Autodesk Inventor part; units mm, degrees
ref_plane "YZ Plane" through (0, 0, 0) normal (1, 0, 0) x (0, 1, 0)
ref_plane "XZ Plane" through (0, 0, 0) normal (0, 1, 0) x (-1, 0, 0)
ref_plane "XY Plane" through (0, 0, 0) normal (0, 0, 1) x (1, 0, 0)
sketch "스케치1" plane through (0, 0, 0) normal (0, 0, 1) x (1, 0, 0)
  line L0 (-3, 27) -> (3, 27)
  line L1 (3, 27) -> (3, -27)
  line L2 (3, -27) -> (-3, -27)
  line L3 (-3, -27) -> (-3, 27)
  point P0 (0, 0)
  dimension "d0" = 6
  dimension "d1" = 54
  dimension "d3" = 3
  dimension "d4" = 27
extrude "돌출1" add sketch "스케치1" along normal blind 4
sketch "스케치2" plane through (0, 0, 4) normal (0, 0, 1) x (1, 0, 0)
  line L0 (3, 27) -> (-3, 27)
  line L1 (-3, 27) -> (-3, -27)
  line L2 (-3, -27) -> (3, -27)
  line L3 (3, -27) -> (3, 27)
  circle A0 centre (0, 24) radius 1.6
  circle A1 centre (0, -24) radius 1.6
  point P0 (0, 0)
  dimension "d7" = 3.2
  dimension "d8" = 3.2
  dimension "d9" = 3
  dimension "d10" = 3
  dimension "d11" = 3
  dimension "d12" = 3
extrude "돌출2" cut sketch "스케치2" against normal up to next contours A0 | A1
chamfer "모따기1" distance 2 angle 45 4 edges at (3, 27, 2) (-3, 27, 2) (-3, -27, 2) (3, -27, 2)
properties part number "큰모터서포터" material "알루미늄 6061"
Can you work these out from the model? Positions are in its coordinate system, mm. Give positions to 0.01 mm unless a question says otherwise; leave off trailing zeros. Loops run counter-clockwise (first coordinate to the right, second up) from the corner with the lowest first, then second, coordinate; pieces in that order, holes last. Notation, with made-up numbers: M 70,54.5 L 96,54.5 A22 cw 96,88.5 Z; hole C -9,41.5 d3. An arc over 180 degrees is marked long. Answer in a Markdown table with one row per item.
1. If I drill on line 1 along Y through (x, z) = (0, 1.3); line 2 along Y through (x, z) = (0.75, 2.35); line 3 along Y through (x, z) = (2.75, 3.3), over which ranges is the centre line in solid material (lowest first)?
Taken from the geometry:
| item | result |
|---|---|
| line 1 | y = -27 to -25.6, -22.4 to 22.4, 25.6 to 27 |
| line 2 | y = -27 to -25.41, -22.59 to 22.59, 25.41 to 27 |
| line 3 | y = -25.25 to 25.25 |
2. For pin 1 Ø2 at (x, y) = (2, -7) entering from -Z, with a flat end and sliding along its axis, tell me the tip position at first contact or that it passes through.
Taken from the geometry:
| item | result |
|---|---|
| pin 1 | stops at z = 0 |
3. Suppose I cut it at A-A on x = 0. Write out the boundary of the cut face in (y, z), plus the area to 3 significant figures.
Taken from the geometry:
| item | result |
|---|---|
| outline | M -27,0 L -25.6,0 L -25.6,4 L -27,4 Z; M -22.4,0 L 22.4,0 L 22.4,4 L -22.4,4 Z; M 25.6,0 L 27,0 L 27,4 L 25.6,4 Z |
| area | 190 mm² |
4. Thinking about a two-plate mould opening in X: for faces 1 (the cylindrical face through (-0.208, 25.586, 2.028)), 2 (the flat face through (0, 0, 0)), 3 (the flat face through (2, 26, 2)), which applies, released by +X, released by -X, zero draft, split by the parting line, or undercut?
Taken from the geometry:
| item | result |
|---|---|
| face 1 | undercut |
| face 2 | zero draft |
| face 3 | released by +X |
5. Suppose I cut it at D-D on x = 2.3. Write out the boundary of the cut face in (y, z).
Taken from the geometry:
| item | result |
|---|---|
| outline | M -25.7,0 L 25.7,0 L 25.7,4 L -25.7,4 Z |
6. Suppose I cut it at B-B on z = 1.25. Write out the boundary of the cut face in (x, y), plus the area to 3 significant figures.
Taken from the geometry:
| item | result |
|---|---|
| outline | M -3,-25 L -1,-27 L 1,-27 L 3,-25 L 3,25 L 1,27 L -1,27 L -3,25 Z; hole C 0,-24 d3.2; hole C 0,24 d3.2 |
| area | 300 mm² |
7. Suppose I cut it at C-C on y = 24. Write out the boundary of the cut face in (x, z).
Taken from the geometry:
| item | result |
|---|---|
| outline | M -3,0 L -1.6,0 L -1.6,4 L -3,4 Z; M 1.6,0 L 3,0 L 3,4 L 1.6,4 Z |
